The listing builds one solid part. Answer for the finished solid, in the listing's coordinates (mm). A direction names the side the tool comes from. Round coordinates to 2 decimals unless told otherwise and drop trailing zeros. Loops run counter-clockwise (first coordinate to the right, second up) from the corner with the lowest first, then second, coordinate; pieces in that order, holes last. Notation, with made-up numbers: (78, 87.5) -> (93, 87.5) arc R30 ccw to (93, 115.5) -> close; hole circle Ø11 at (-31.75, 89). An arc over 180 degrees is marked (long way). Use a Markdown table: item, result. Add a question column.
Q1. Section B-B on y = 14 is taken. Give the vertices of the cut face in (x, z).
Q2. Consider line 1 (Y direction, x = 0, z = -0.6); line 2 (X direction, y = -8, z = -19.5); line 3 (Y direction, x = -7, z = 15.5). Determine where each line is inside the solid, lowest interval first.
Q3. Given pin 1 Ø2 at (x, z) = (-7.5, -14) entering from -Y; pin 2 Ø2 at (x, z) = (-13, -19) entering from -Y; pin 3 Ø1.3 at (x, y) = (0, 27) entering from +Z, each flat-ended and moving along its own axis, determine where each tip first touches the part or whether it passes through.
Q4. For a pull along X with two mould halves and no side action, classify faces 3 (the cylindrical face through (0, 28, 0)), 4 (the flat face through (3.5, 28, 0)), 5 (the cylindrical face through (0.1, 33.5, 0)), 6 (the flat face through (-3.5, 28, 0)) as released by +X, released by -X, zero draft, split by the parting line, or undercut.
Q5. Which of the six approach directions +Z, -Z, +X, -X, +Y, -Y give full straight-line access (tool end or side, diameter ignored) to faces 1 (the flat face through (0, 26.7, 2.5)), 2 (the flat face through (0, 26.7, -2.5))?
Q6. Section A-A on z = -10 is taken. Give the vertices of the cut face in (x, y), then the cut area to 3 significant figures.
from build123d import *

# Parameters (mm, degrees)
SKETCH2_R           = 2
BOSS_EXTRUDE1_DEPTH = 2.5
FILLET1_R           = 1


with BuildPart() as part:
    # Sketch1 → Revolve1 (revolve)
    with BuildSketch(Plane(origin=(0, 0, 0), x_dir=(1, 0, 0), z_dir=(0, 1, 0))):
        with BuildLine():
            Line((-25, 0), (25, 0))
            ThreePointArc((25, 0), (0, 25), (-25, 0))
        make_face()
    revolve(axis=Axis((-25, 0, 0), (1, 0, 0)))

    # Sketch2 → Boss-Extrude1 (add, symmetric)
    with BuildSketch(Plane.XY):
        with BuildLine():
            Line((-3.5, 20), (3.5, 20))
            Line((3.5, 20), (3.5, 30))
            ThreePointArc((3.5, 30), (0, 33.5), (-3.5, 30))
            Line((-3.5, 30), (-3.5, 20))
        make_face()
        with Locations((0, 30)):
            Circle(SKETCH2_R, mode=Mode.SUBTRACT)
    extrude(amount=BOSS_EXTRUDE1_DEPTH, both=True)

    # Fillet1
    fillet1_edges = [part.edges().sort_by_distance(p)[0] for p in [
        (-3.5, 27.313610356, 2.5),
        (3.5, 27.313610356, 2.5),
        (0, 33.5, 2.5),
    ]]
    fillet(fillet1_edges, radius=FILLET1_R)
    fillet1_2_edges = [part.edges().sort_by_distance(p)[0] for p in [
        (-3.5, 27.313610356, -2.5),
        (0, 33.5, -2.5),
        (3.5, 27.313610356, -2.5),
    ]]
    fillet(fillet1_2_edges, radius=FILLET1_R)
    fillet1_3_edges = [part.edges().sort_by_distance(p)[0] for p in [
        (0, 24.874685928, -2.5),
    ]]
    fillet(fillet1_3_edges, radius=FILLET1_R)
    # the kernel refuses this fillet: 1 mm, written as the material it takes off along each edge
    with BuildSketch(Plane(origin=(0, 30, -2.5), x_dir=(1, 0, 0), z_dir=(0, -1, 0))) as fillet1_4_piece_1:
        with BuildLine():
            CenterArc((2 + FILLET1_R, FILLET1_R), FILLET1_R, 180, 90)
            Line((2, FILLET1_R), (2 - FILLET1_R * 0.02, FILLET1_R))
            Line((2 - FILLET1_R * 0.02, FILLET1_R), (2 - FILLET1_R * 0.02, -FILLET1_R * 0.02))
            Line((2 - FILLET1_R * 0.02, -FILLET1_R * 0.02), (2 + FILLET1_R, -FILLET1_R * 0.02))
            Line((2 + FILLET1_R, -FILLET1_R * 0.02), (2 + FILLET1_R, 0))
        make_face()
    revolve(axis=Axis((0, 30, -2.5), (0, 0, 1)), mode=Mode.SUBTRACT)
    # the kernel refuses this fillet: 1 mm, written as the material it takes off along each edge
    with BuildSketch(Plane(origin=(0, 30, 2.5), x_dir=(1, 0, 0), z_dir=(0, -1, 0))) as fillet1_5_piece_1:
        with BuildLine():
            CenterArc((2 + FILLET1_R, -FILLET1_R), FILLET1_R, 90, 90)
            Line((2, -FILLET1_R), (2 - FILLET1_R * 0.02, -FILLET1_R))
            Line((2 - FILLET1_R * 0.02, -FILLET1_R), (2 - FILLET1_R * 0.02, FILLET1_R * 0.02))
            Line((2 - FILLET1_R * 0.02, FILLET1_R * 0.02), (2 + FILLET1_R, FILLET1_R * 0.02))
            Line((2 + FILLET1_R, FILLET1_R * 0.02), (2 + FILLET1_R, 0))
        make_face()
    revolve(axis=Axis((0, 30, 2.5), (0, 0, 1)), mode=Mode.SUBTRACT)


solid = part.part
Checked values:
| question | item | result |
|---|---|---|
| 1 | outline | circle Ø41.42 at (0, 0) |
| 2 | line 1 | y = -24.99 to 28, 32 to 33.5 |
| 2 | line 2 | x = -13.44 to 13.44 |
| 2 | line 3 | y = -18.32 to 18.32 |
| 3 | pin 1 | stops at y = -20.09 |
| 3 | pin 2 | stops at y = -11.83 |
| 3 | pin 3 | stops at z = 2.5 |
| 4 | face 3 | undercut |
| 4 | face 4 | released by +X |
| 4 | face 5 | split by the parting line |
| 4 | face 6 | released by -X |
| 5 | face 1 | +Z, +X, -X, +Y |
| 5 | face 2 | -Z, +X, -X, +Y |
| 6 | outline | circle Ø45.83 at (0, 0) |
| 6 | area | 1,650 mm2 |
